from build123d import *

# Parameters (mm, degrees)
SKETCH_1_R          = 6.5
SKETCH_1_R_2        = 1.5
SKETCH_1_W          = 15
SKETCH_1_H          = 12
EXTRUDE_1_DEPTH     = 5
HOLE_WIZARD_M3_1_D  = 2.5
SKETCH_2_W          = 9
SKETCH_2_H          = 83.78955867
CUT_EXTRUDE_1_DEPTH = 1
FILLET_1_R          = 3
EXTRUDE_2_DEPTH     = 2
CHAMFER_1_SIZE      = 2
SKETCH_5_R          = 1.5
EXTRUDE_4_DEPTH     = 5
FILLET_2_R          = 5
EXTRUDE_START       = 2
SKETCH_6_R          = 3
SKETCH_6_R_2        = 1.5
EXTRUDE_5_DEPTH     = 2


with BuildPart() as part:
    # 草图1 → 凸台-拉伸1 (new body)
    with BuildSketch(Plane.XY):
        Polygon((6, 55), (-6, 55), (-15, 35), (-15, 31), (-8, -16), (8, -16), (15, 31), (15, 35), align=None)
        Circle(SKETCH_1_R, mode=Mode.SUBTRACT)
        with Locations((0, 49)):
            Circle(SKETCH_1_R_2, mode=Mode.SUBTRACT)
        with Locations((-8, 40)):
            Circle(SKETCH_1_R_2, mode=Mode.SUBTRACT)
        with Locations(Location((8, 40, 0), (0, 0, 180))):
            Circle(SKETCH_1_R_2, mode=Mode.SUBTRACT)
        with Locations((0, 19)):
            Rectangle(SKETCH_1_W, SKETCH_1_H, mode=Mode.SUBTRACT)
    extrude(amount=EXTRUDE_1_DEPTH)

    # M3 螺纹孔1 (through all)
    with Locations(Plane.XY.offset(5)):
        with Locations((0, 29), (0, 9), (0, -11)):
            Hole(HOLE_WIZARD_M3_1_D / 2)

    # 草图2 → 切除-拉伸1 (cut)
    with BuildSketch(Plane.XY.offset(5)):
        with Locations((0, 22.915271632)):
            Rectangle(SKETCH_2_W, SKETCH_2_H)
    extrude(amount=-CUT_EXTRUDE_1_DEPTH, mode=Mode.SUBTRACT)

    # 圆角1
    fillet_1_edges = [part.edges().sort_by_distance(p)[0] for p in [
        (7.5, 13, 2.5),
        (-7.5, 13, 2.5),
        (-7.5, 25, 2.5),
        (7.5, 25, 2.5),
    ]]
    fillet(fillet_1_edges, radius=FILLET_1_R)

    # 草图4 → 凸台-拉伸2 (add)
    with BuildSketch(Plane.XY.offset(5)):
        Polygon((-8, -16), (-4.5, -16), (-4.5, -14), (-8.29787234, -14), align=None)
        Polygon((4.5, -14), (8.29787234, -14), (8, -16), (4.5, -16), align=None)
    extrude(amount=EXTRUDE_2_DEPTH)

    # 倒角1
    chamfer_1_edges = [part.edges().sort_by_distance(p)[0] for p in [
        (-9.5, 40, 5),
        (9.5, 40, 5),
    ]]
    chamfer(chamfer_1_edges, length=CHAMFER_1_SIZE - 0.0001)  # a hair under: the kernel refuses the full size

    # 草图5 → 凸台-拉伸4 (add)
    with BuildSketch(Plane.XY.offset(5)):
        with BuildLine():
            Line((6, 55), (13.5, 55))
            ThreePointArc((13.5, 55), (18.049597051, 47.926074574), (9.725789999, 46.720466669))
            Line((9.725789999, 46.720466669), (6, 55))
        make_face()
        with Locations((13.5, 50)):
            Circle(SKETCH_5_R, mode=Mode.SUBTRACT)
    extrude(amount=-EXTRUDE_4_DEPTH)

    # 圆角2
    fillet_2_edges = [part.edges().sort_by_distance(p)[0] for p in [
        (9.725789999, 46.720466669, 2.5),
    ]]
    fillet(fillet_2_edges, radius=FILLET_2_R)

    # 草图6 → 凸台-拉伸5 (add)
    with BuildSketch(Plane.XY.offset(5).offset(EXTRUDE_START)):
        with Locations((13.5, 50)):
            Circle(SKETCH_6_R)
        with Locations((13.5, 50)):
            Circle(SKETCH_6_R_2, mode=Mode.SUBTRACT)
    extrude(amount=-EXTRUDE_5_DEPTH)


with BuildPart() as body_2:
    # 镜向1: mirrored copy
    add(part.part.mirror(Plane(origin=(0, 0, 0), x_dir=(0, 0, 1), z_dir=(1, 0, 0))))


solid = body_2.part
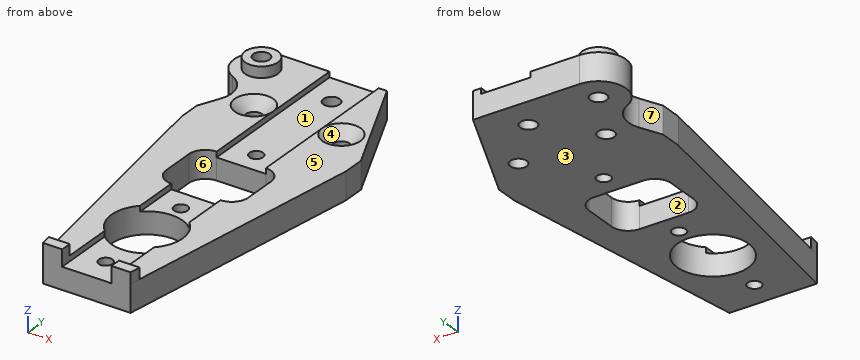
Here's how the part is built. I have some questions about the finished solid (model axes, mm). Face numbers are marked on the shaded views. A direction names the side the tool comes from. Coordinates: 2 decimals unless noted, no trailing zeros. Write each loop counter-clockwise with the first axis right and the second up, starting at its lowest first coordinate (ties: lowest second). Pieces come first, ordered by that corner, then holes.
Item 1: Will these pins go through, and if not, where does the flat tip stop? pin 1 (3 mm diameter, centred on x = 8, y = 8.5, fed in from +Z); pin 2 (0.6 mm diameter, centred on x = -7, z = 6, fed in from +Y); pin 3 (4 mm diameter, centred on y = -8.5, z = 6, fed in from -X) (3 decimals).
Item 2: I want a section at B-B on z = 1. Count the separate pieces of the cut face and the enclosed holes in it, and give its area (3 significant figures).
Item 3: I want a section at A-A on z = 5.75. Write out the boundary of the cut face in (x, y), and give its area (3 significant figures).
Item 4: If I drill on line 1 (Z direction, x = -5.5, y = 26.5); line 2 (Z direction, x = 2.5, y = 8); line 3 (X direction, y = 5, z = 1.5), over which ranges is the centre line in solid material (lowest first)?
Item 5: If we mould it in two halves opening along X, with no side actions, what happens to the marked faces 4, 5, 6 and 7? For each: +X half, -X half, draft (parallel to the pull), parting line (faces both ways), or undercut.
Item 6: On a 3-axis mill with a long thin cutter (end or side, diameter ignored), from which of +Z, -Z, +X, -X, +Y, -Y can I reach the whole of each face in a straight line? I mean the marked faces 1, 2 and 3. Say none if no direction works.
Item 7: I want a section at C-C on y = 29. Write out the boundary of the cut face in (x, z).
Item 8: I want a section at D-D on y = 19.5. Write out the boundary of the cut face in (x, z), and give its area (3 significant figures).
Findings below:
1. pin 1: stops at z = 5
1. pin 2: stops at y = -14
1. pin 3: stops at x = -9.375
2. separate pieces: 1
2. enclosed holes: 9
2. area: 1,370 mm2
3. outline: circle Ø6 at (-13.5, 50); (-8.3, -14) - (-8, -16) - (-4.5, -16) - (-4.5, -14) - close; (4.5, -16) - (8, -16) - (8.3, -14) - (4.5, -14) - close; hole circle Ø3 at (-13.5, 50)
3. area: 35.8 mm2
4. line 1: z = 0 to 5
4. line 2: z = 0 to 4
4. line 3: x = -11.13 to -4.15, 4.15 to 11.13
5. face 4: undercut
5. face 5: draft
5. face 6: undercut
5. face 7: -X half
6. face 1: +Z, +Y, -Y
6. face 2: +Z, -Z
6. face 3: -Z, +X, -X, +Y, -Y
7. outline: (-14.7, 0) - (-1.25, 0) - (-1.25, 4) - (-4.5, 4) - (-4.5, 5) - (-14.7, 5) - close; (1.25, 0) - (14.7, 0) - (14.7, 5) - (4.5, 5) - (4.5, 4) - (1.25, 4) - close
8. outline: (-13.29, 0) - (-7.5, 0) - (-7.5, 5) - (-13.29, 5) - close; (7.5, 0) - (13.29, 0) - (13.29, 5) - (7.5, 5) - close
8. area: 57.9 mm2
